Print and shaded views of the part. All mm, measured from the part's lowest x, y and z. A direction names the side the tool comes from. Coordinates: 2 decimals unless noted, no trailing zeros. Order: outer loops, then holes, each group sorted by start corner. A loop starts at its lowest first (then second) coordinate and runs counter-clockwise, first axis right, second up. Notation, with made-up numbers: M 70.5,30.25 L 107.5,30.25 A17 cw 107.5,50.25 Z; hole C -4,55 d5. An arc over 180 degrees is marked long. Use a Markdown table: item, result. Add a question column.
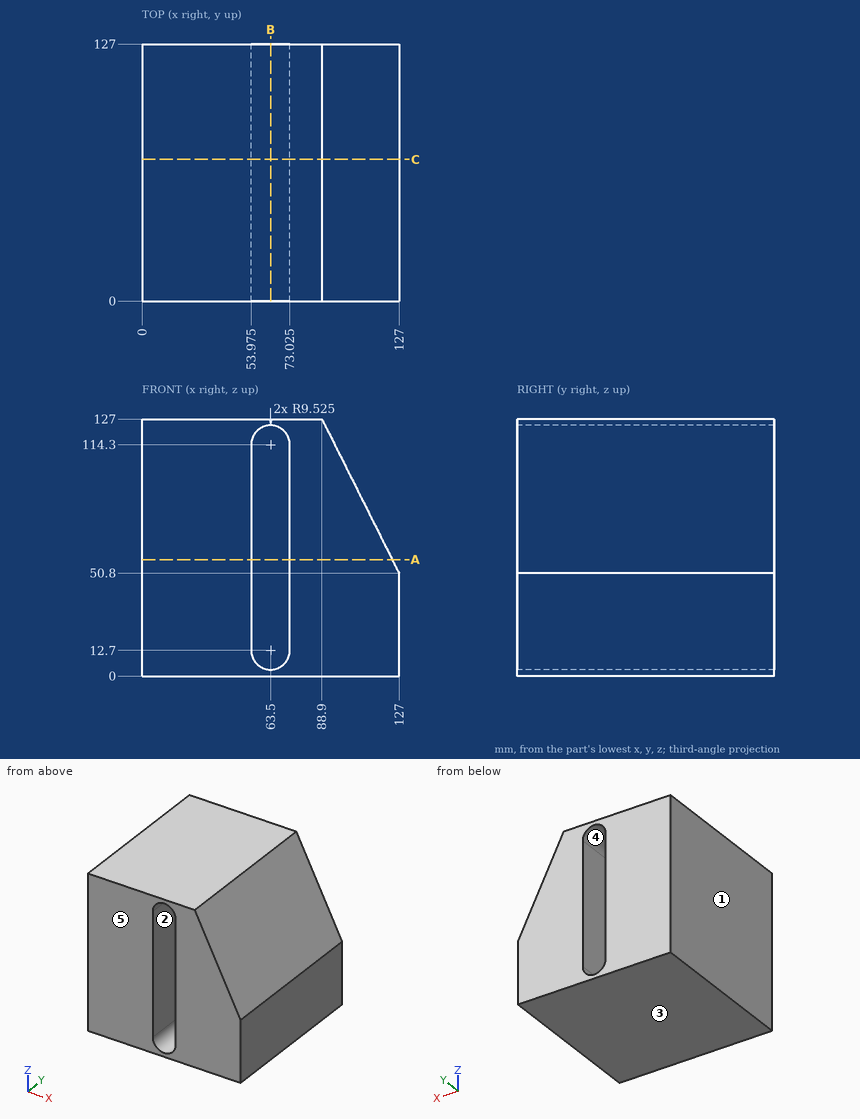
(1) Mould opens along Z. For the marked faces 3, 4 and 5 say: released by +Z, released by -Z, zero draft, split by the parting line, or undercut.
(2) Drill centre lines: line 1 along X through (y, z) = (26, 48) (3 decimals); line 2 along X through (y, z) = (34.5, 112) (3 decimals); line 3 along Z through (x, y) = (66.5, 107.5). Where is each one in solid material? Low to high. Write a range as from..to.
(3) Slice it at B-B on x = 63.5. Give the cut face in (y, z) (3 decimals), and give its area (3 significant figures).
(4) Slice it at A-A on z = 57.5. Give the cut face in (x, y) (3 decimals), and give its area (3 significant figures).
(5) Which spindle directions (+Z, -Z, +X, -X, +Y, -Y) get a long thin tool onto all of the face, cutting with end or side? Do the marked faces 1 and 2. Say none if no direction does.
(6) Slice it at C-C on y = 70. Give the cut face in (x, z) (3 decimals).
(7) Drop flat-ended pins along their axis: P1, Ø3, axis at x = 56, z = 36.5, coming from the -Y side; P2, Ø8, axis at y = 55, z = 94.5, coming from the +X side. Give the stop position or say it passes through.
Solutions:
| question | item | result |
|---|---|---|
| 1 | face 3 | released by -Z |
| 1 | face 4 | undercut |
| 1 | face 5 | zero draft |
| 2 | line 1 | 0..53.975, 73.025..127 |
| 2 | line 2 | 0..53.975, 73.025..96.4 |
| 2 | line 3 | 0..3.66, 123.34..127 |
| 3 | outline | M 0,0 L 127,0 L 127,3.175 L 0,3.175 Z; M 0,123.825 L 127,123.825 L 127,127 L 0,127 Z |
| 3 | area | 806 mm² |
| 4 | outline | M 0,0 L 53.975,0 L 53.975,127 L 0,127 Z; M 73.025,0 L 123.65,0 L 123.65,127 L 73.025,127 Z |
| 4 | area | 13,300 mm² |
| 5 | face 1 | +Z, -Z, -X, +Y, -Y |
| 5 | face 2 | +Y, -Y |
| 6 | outline | M 0,0 L 127,0 L 127,50.8 L 88.9,127 L 0,127 Z; hole M 53.975,12.7 A9.525 ccw 73.025,12.7 L 73.025,114.3 A9.525 ccw 53.975,114.3 Z |
| 7 | P1 | through |
| 7 | P2 | x = 107.15 |
